Check sheet for the modelled part. Datum: model origin and axes. Units: mm. Face numbers are marked on the shaded views. A direction names the side the tool comes from. Give positions to 0.01 mm unless a question says otherwise; leave off trailing zeros. Loops run counter-clockwise (first coordinate to the right, second up) from the corner with the lowest first, then second, coordinate; pieces in that order, holes last. Notation, with made-up numbers: (40, 67) -> (45, 67) arc R10 cw to (45, 72) -> close; hole circle Ø3 at (17, 50). An arc over 180 degrees is marked (long way). Write each question's results on one line, items separated by ' | '. Start each with the question number.
1. Tool access check on the marked faces 1, 2 and 3. Record the directions out of +Z, -Z, +X, -X, +Y, -Y that give a thin tool (end or side, any length) a straight path to the whole face; none if there is none.
2. Material ranges on L1, parallel to Y at x = 0, z = 3.25; L2, parallel to Z at x = -2, y = 7; L3, parallel to X at y = -10.5, z = 5, recorded low to high. Write a range as from..to.
3. Cross-section at B-B on x = 0. Record the boundary of the cut face in (y, z).
4. Cross-section at C-C on y = 27. Record the boundary of the cut face in (x, z), and give its area (3 significant figures).
5. Gauge pin test, flat ends, axial feed: pin 1 Ø1.5 at (y, z) = (-3, -4) entering from +X; pin 2 Ø10 at (y, z) = (-0.5, -0.5) entering from -X; pin 3 Ø2 at (x, y) = (3.5, 48.5) entering from +Z. Record the tip position at first contact, or that the pin passes through.
6. Cross-section at A-A on z = 0. Record the boundary of the cut face in (x, y), and give its area (3 significant figures).
7. Cross-section at D-D on y = -19. Record the boundary of the cut face in (x, z).
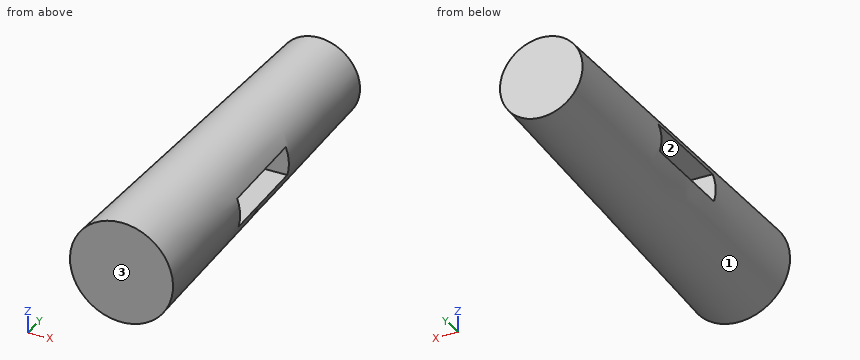
from build123d import *

# Parameters (mm, degrees)
CUT_EXTRUDE1_DEPTH      = 67.746531734
CUT_EXTRUDE1_DEPTH_BACK = 67.746531734
SKETCH3_W               = 7
SKETCH3_H               = 24


with BuildPart() as part:
    # Sketch2 → Revolve1 (revolve)
    with BuildSketch(Plane.XY, mode=Mode.PRIVATE) as revolve1_sk:
        Polygon((0, 64.324019608), (10.1, 64.324019608), (12.6, -27.675980392), (0, -27.675980392), align=None)
    revolve(revolve1_sk.sketch.rotate(Axis((0, 86.777607614, 0), (0, -1, 0)), 90), axis=Axis((0, 86.777607614, 0), (0, -1, 0)))

    # Sketch3 → Cut-Extrude1 (cut, two sides: drawn at the far end of the back side and taken through both)
    with BuildSketch(Plane(origin=(0, 0, 0), x_dir=(0, 0, -1), z_dir=(1, 0, 0)).offset(-CUT_EXTRUDE1_DEPTH_BACK)):
        with Locations((-0.559695247, 17.324019608)):
            Rectangle(SKETCH3_W, SKETCH3_H)
    extrude(amount=CUT_EXTRUDE1_DEPTH + CUT_EXTRUDE1_DEPTH_BACK, mode=Mode.SUBTRACT)


solid = part.part
Geometry says:
1) face 1: +Y | face 2: +X, -X | face 3: +Z, -Z, +X, -X, -Y
2) L1: -27.68..5.32, 29.32..64.32 | L2: -11.48..-2.94, 4.06..11.48 | L3: -11.06..11.06
3) outline: (-27.68, -12.6) -> (64.32, -10.1) -> (64.32, 10.1) -> (-27.68, 12.6) -> close; hole (5.32, -2.94) -> (29.32, -2.94) -> (29.32, 4.06) -> (5.32, 4.06) -> close
4) outline: (-10.72, -2.94) arc R11.11 ccw to (10.72, -2.94) -> close; (-10.35, 4.06) -> (10.35, 4.06) arc R11.11 ccw to start | area: 235 mm^2
5) pin 1: x = 11.48 | pin 2: x = -12 | pin 3: z = 10.23
6) outline: (-12.6, -27.68) -> (12.6, -27.68) -> (11.7, 5.32) -> (-11.7, 5.32) -> close; (-11.05, 29.32) -> (11.05, 29.32) -> (10.1, 64.32) -> (-10.1, 64.32) -> close | area: 1,540 mm^2
7) outline: circle Ø24.73 at (0, 0)
